from build123d import *

# Parameters (mm, degrees)
SKETCH1_R           = 1.5
BOSS_EXTRUDE1_DEPTH = 3


with BuildPart() as part:
    # Sketch1 → Boss-Extrude1 (new body)
    with BuildSketch(Plane(origin=(0, 0, 0), x_dir=(1, 0, 0), z_dir=(0, 1, 0))):
        Polygon((-37.889024654, 3.81895344), (-27.889024654, 3.81895344), (-27.889024654, 0.81895344), (-20.889024654, 0.81895344), (-20.889024654, -7.98104656), (-1.629024654, -7.98104656), (-6.329024654, -12.68104656), (-45.889024654, -12.68104656), (-45.889024654, -8.18104656), (-48.889024654, -8.18104656), (-48.889024654, -3.18104656), (-45.889024654, -3.18104656), (-45.889024654, 0.81895344), (-37.889024654, 0.81895344), align=None)
        with Locations((-26.889024654, -7.18104656)):
            Circle(SKETCH1_R, mode=Mode.SUBTRACT)
    extrude(amount=BOSS_EXTRUDE1_DEPTH)


solid = part.part
CAD build for the part. Positions are in the model's coordinates, mm. A direction names the side the tool comes from. Round coordinates to 2 decimals unless told otherwise and drop trailing zeros. Write each loop counter-clockwise with the first axis right and the second up, starting at its lowest first coordinate (ties: lowest second). Pieces come first, ordered by that corner, then holes. Notation, with made-up numbers: M -26,-28.75 L 4,-28.75 A9 ccw 4,-20.75 Z; hole C 85.25,15.5 d6. An arc over 180 degrees is marked long. Use a Markdown table: item, result. Add a question column.
1. Drill centre lines: probe 1 along X at (y, z) = (2.55, 7); probe 2 along Z at (x, y) = (-41, 2.65); probe 3 along Z at (x, y) = (-20, 1.35). Where is each one in solid material? Low to high.
2. Slice it at B-B on y = 0.6. Give the cut face in (x, z), then the cut area to 3 significant figures.
3. Slice it at C-C on z = 4. Give the cut face in (x, y), then the cut area to 3 significant figures.
4. Pull direction X, two halves, no side cores. Call faces 5 (the face through (-27.995, 1.479, 6.167)), 6 (the face through (-20.889, 1, 4)), 7 (the face through (-48.889, 1, 6)), 8 (the face through (-30, 0, 6)): released by +X, released by -X, zero draft, split by the parting line, or undercut.
5. 3-axis set-ups, long thin cutter, end or side, ignore diameter. For faces 1 (the face through (-3.95, 1.48, 10.3)), 2 (the face through (-47, 1, 8.181)), 3 (the face through (-27.889, 1, -2)), 4 (the face through (-47, 1, 3.181)): which of +Z, -Z, +X, -X, +Y, -Y reach the whole face in a straight line?
6. Flat gauge pins, fed straight in: P1, Ø0.9, axis at y = 1.5, z = -1.5, coming from the +X side; P2, Ø1.5, axis at y = 1, z = 1.5, coming from the -X side; P3, Ø1, axis at x = -16, y = 2.5, coming from the -Z side. Where does each tip first touch, or does it go through?
7. Slice it at A-A on x = -27. Give the cut face in (y, z), then the cut area to 3 significant figures.
8. Slice it at D-D on x = -10. Give the cut face in (y, z), then the cut area to 3 significant figures.
Reply:
| question | item | result |
|---|---|---|
| 1 | probe 1 | x = -48.89 to -28.38, -25.4 to -20.89 |
| 1 | probe 2 | z = -0.82 to 12.68 |
| 1 | probe 3 | z = 7.98 to 12.68 |
| 2 | outline | M -48.89,3.18 L -45.89,3.18 L -45.89,-0.82 L -37.89,-0.82 L -37.89,-3.82 L -27.89,-3.82 L -27.89,-0.82 L -20.89,-0.82 L -20.89,7.98 L -1.63,7.98 L -6.33,12.68 L -45.89,12.68 L -45.89,8.18 L -48.89,8.18 Z; hole C -26.89,7.18 d3 |
| 2 | area | 455 mm^2 |
| 3 | outline | M -48.89,0 L -20.89,0 L -20.89,3 L -48.89,3 Z |
| 3 | area | 84.0 mm^2 |
| 4 | face 5 | undercut |
| 4 | face 6 | released by +X |
| 4 | face 7 | released by -X |
| 4 | face 8 | zero draft |
| 5 | face 1 | +Z, +X, +Y, -Y |
| 5 | face 2 | +Z, -X, +Y, -Y |
| 5 | face 3 | -Z, +X, +Y, -Y |
| 5 | face 4 | -Z, -X, +Y, -Y |
| 6 | P1 | stops at x = -27.89 |
| 6 | P2 | stops at x = -45.89 |
| 6 | P3 | stops at z = 7.98 |
| 7 | outline | M 0,-0.82 L 3,-0.82 L 3,5.69 L 0,5.69 Z; M 0,8.68 L 3,8.68 L 3,12.68 L 0,12.68 Z |
| 7 | area | 31.5 mm^2 |
| 8 | outline | M 0,7.98 L 3,7.98 L 3,12.68 L 0,12.68 Z |
| 8 | area | 14.1 mm^2 |
